from build123d import *

# Parameters (mm, degrees)
SKETCH1_R           = 8
BOSS_EXTRUDE1_DEPTH = 880
SKETCH4_R           = 2.1
CUT_EXTRUDE2_DEPTH  = 12.4
LPATTERN1_COUNT     = 5
LPATTERN1_PITCH     = 150


with BuildPart() as part:
    # Sketch1 → Boss-Extrude1 (new body)
    with BuildSketch(Plane.XY):
        Circle(SKETCH1_R)
    extrude(amount=BOSS_EXTRUDE1_DEPTH)

    # Sketch4 → Cut-Extrude2 (cut)
    with BuildSketch(Plane(origin=(0, -8, 0), x_dir=(-1, 0, 0), z_dir=(0, 1, 0))):
        with Locations(Location((0, 100, 0), (0, 0, 270))):
            Circle(SKETCH4_R)
    cut_extrude2 = extrude(amount=CUT_EXTRUDE2_DEPTH, mode=Mode.SUBTRACT)

    # LPattern1: Cut-Extrude2 ×5
    with Locations(*[(0, 0, i * LPATTERN1_PITCH) for i in range(1, LPATTERN1_COUNT)]):
        add(cut_extrude2, mode=Mode.SUBTRACT)


solid = part.part
Design review of the part built by this model. Coordinates are the model's own, in mm. Coordinates: 2 decimals unless noted, no trailing zeros. Loops run counter-clockwise (first coordinate to the right, second up) from the corner with the lowest first, then second, coordinate; pieces in that order, holes last. Notation, with made-up numbers: M 84.25,58.25 L 94.25,58.25 A13 cw 94.25,64.25 Z; hole C 72.25,4 d5. An arc over 180 degrees is marked long. Use one line per item in the form item = value.
(1) Consider section B-B (z = 678). Write out the cut boundary in (x, y).
Return value:
outline = C 0,0 d16
(2) Consider section A-A (y = -4.25). Write out the cut boundary in (x, z), and give its area (3 significant figures).
Return value:
outline = M -6.78,0 L 6.78,0 L 6.78,880 L -6.78,880 Z; hole C 0,100 d4.2; hole C 0,250 d4.2; hole C 0,400 d4.2; hole C 0,550 d4.2; hole C 0,700 d4.2
area = 11,900 mm2
(3) For line 1 along X through (y, z) = (0.75, 250); line 2 along X through (y, z) = (-1.5, 494.5); line 3 along X through (y, z) = (-3.25, 250), list the stretches that pass through material, from the lowest coordinate up. Write a range as from..to.
Return value:
line_1 = -7.96..-2.1, 2.1..7.96
line_2 = -7.86..7.86
line_3 = -7.31..-2.1, 2.1..7.31
(4) Clearance check with flat-ended pins moving along their axes: P1, Ø5, axis at x = 2, z = 528, coming from the +Y side; P2, Ø2.5, axis at x = 0, z = 400, coming from the -Y side; P3, Ø4.5, axis at x = -1, z = 700, coming from the -Y side; P4, Ø6, axis at x = 6, z = 661, coming from the +Y side. State where each tip first meets the part, or that it passes through.
Return value:
P1 = 8
P2 = 4.4
P3 = -8
P4 = 7.42
(5) Consider section C-C (x = -5). Write out the cut boundary in (y, z) (3 decimals).
Return value:
outline = M -6.245,0 L 6.245,0 L 6.245,880 L -6.245,880 Z
